Answer from the drawing. Dimensions are ordinates in mm from the lowest x, y and z of the part. A direction names the side the tool comes from. Coordinates: 2 decimals unless noted, no trailing zeros. Order: outer loops, then holes, each group sorted by start corner. A loop starts at its lowest first (then second) coordinate and runs counter-clockwise, first axis right, second up. Notation, with made-up numbers: (9.5, 69.25) - (67.5, 69.25) arc R14 cw to (67.5, 96.25) - close; hole circle Ø9 at (12.25, -8). An arc over 180 degrees is marked (long way). Answer as a JSON object with one key per item and string values. Group by question number.
1) Find the intervals of material crossed by line 1 along Y through (x, z) = (10, 5.5); line 2 along Y through (x, z) = (10, 9.55); line 3 along X through (y, z) = (15, 6), in increasing order.
2) Section B-B (y = 35) is taken. Give the vertices of the cut face in (x, z).
3) A tool of negligible diameter and unlimited length cuts with its end or side. For the marked faces 1 and 2, from which of +Z, -Z, +X, -X, +Y, -Y can it reach the whole face along a straight path? Write none if from no direction.
4) The mould has two halves that part along Y. Classify the marked faces 3, 4, 5 and 6: released by +Y, released by -Y, zero draft, split by the parting line, or undercut.
5) Section C-C (x = 45) is taken. Give the vertices of the cut face in (y, z).
6) Section A-A (x = 80) is taken. Give the vertices of the cut face in (y, z), plus the area to 3 significant figures.
7) Section D-D (z = 5) is taken. Give the vertices of the cut face in (x, y).
8) Each of these flat-tipped pins is pushed along its axis until it touches: P1, Ø4, axis at x = 9, y = 14, coming from the +Z side; P2, Ø3, axis at x = 60.5, z = 4.5, coming from the -Y side; P3, Ø4, axis at x = 3, z = 2.5, coming from the -Y side; P4, Ø2.5, axis at x = 87, z = 5.5, coming from the +Y side. Where does it stop, or does it pass through?
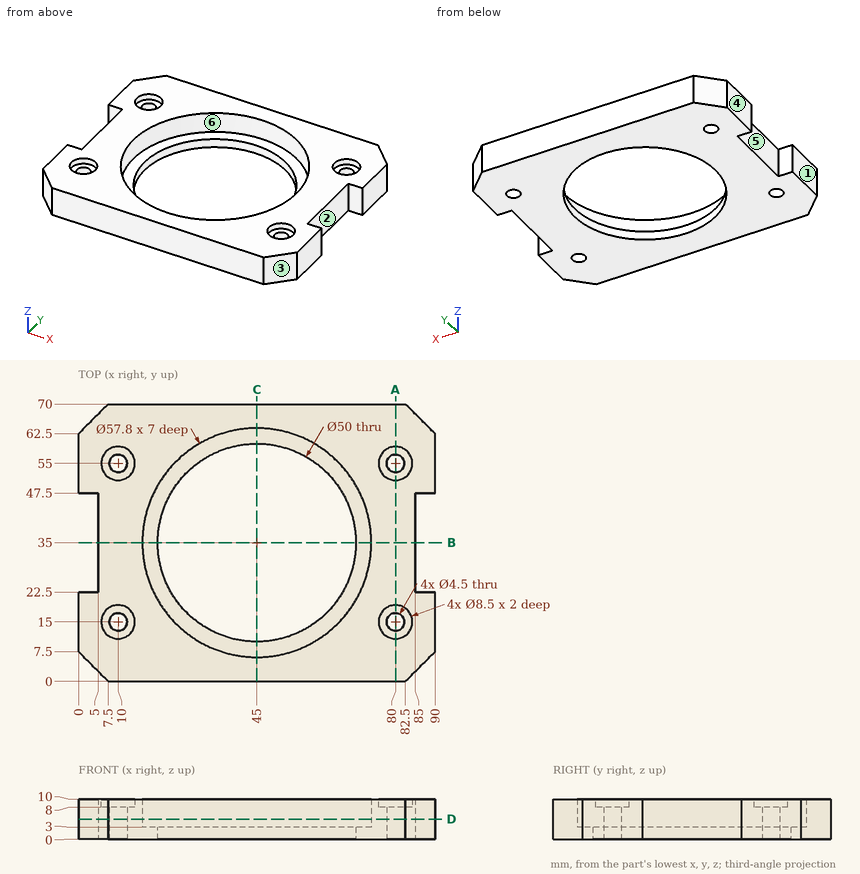
Report:
{
 "1": {"line 1": "y = 0 to 12.75, 17.25 to 52.75, 57.25 to 70", "line 2": "y = 0 to 10.75, 19.25 to 50.75, 59.25 to 70", "line 3": "x = 0 to 7.75, 12.25 to 24.14, 65.86 to 77.75, 82.25 to 90"},
 "2": {"outline": "(5, 0) - (20, 0) - (20, 3) - (16.1, 3) - (16.1, 10) - (5, 10) - close; (70, 0) - (85, 0) - (85, 10) - (73.9, 10) - (73.9, 3) - (70, 3) - close"},
 "3": {"face 1": "+Z, -Z, -X, +Y, -Y", "face 2": "+Z, -Z, +X"},
 "4": {"face 3": "released by -Y", "face 4": "zero draft", "face 5": "undercut", "face 6": "undercut"},
 "5": {"outline": "(0, 0) - (10, 0) - (10, 3) - (6.1, 3) - (6.1, 10) - (0, 10) - close; (60, 0) - (70, 0) - (70, 10) - (63.9, 10) - (63.9, 3) - (60, 3) - close"},
 "6": {"outline": "(0, 0) - (12.75, 0) - (12.75, 8) - (10.75, 8) - (10.75, 10) - (0, 10) - close; (17.25, 0) - (52.75, 0) - (52.75, 8) - (50.75, 8) - (50.75, 10) - (19.25, 10) - (19.25, 8) - (17.25, 8) - close; (57.25, 0) - (70, 0) - (70, 10) - (59.25, 10) - (59.25, 8) - (57.25, 8) - close", "area": "594 mm²"},
 "7": {"outline": "(0, 7.5) - (7.5, 0) - (82.5, 0) - (90, 7.5) - (90, 22.5) - (85, 22.5) - (85, 47.5) - (90, 47.5) - (90, 62.5) - (82.5, 70) - (7.5, 70) - (0, 62.5) - (0, 47.5) - (5, 47.5) - (5, 22.5) - (0, 22.5) - close; hole circle Ø4.5 at (10, 15); hole circle Ø4.5 at (10, 55); hole circle Ø57.8 at (45, 35); hole circle Ø4.5 at (80, 15); hole circle Ø4.5 at (80, 55)"},
 "8": {"P1": "stops at z = 8", "P2": "stops at y = 0", "P3": "stops at y = 2.5", "P4": "stops at y = 66.75"}
}
